Here's how the part is built. I have some questions about the finished solid (model axes, mm). Coordinates: 2 decimals unless noted, no trailing zeros. Write each loop counter-clockwise with the first axis right and the second up, starting at its lowest first coordinate (ties: lowest second). Pieces come first, ordered by that corner, then holes.
Item 1: If I drill on line 1 (Y direction, x = 50, z = 1.65); line 2 (Y direction, x = 68.5, z = 2.95); line 3 (Y direction, x = 30.5, z = 1.3), over which ranges is the centre line in solid material (lowest first)?
Item 2: If we section it at A-A (x = 26): Please give me the cut outline in (y, z) (3 decimals).
Item 3: If we section it at B-B (y = 26.5): Please give me the cut outline in (x, z) (3 decimals), then the cut area to 3 significant figures.
Item 4: We'd pull the mould along X, two halves only. Please class faces 1 (the face through (32.355, 36.9, 1.565)), 2 (the face through (48, 43, 0)): +X half, -X half, draft (parallel to the pull), parting line (faces both ways), or undercut.
Item 5: If we section it at C-C (y = 76): Please give me the cut outline in (x, z) (1 decimal), then the cut area to 3 significant figures.
Item 6: I'm going to push flat-ended pins straight in: pin 1 Ø0.6 at (x, z) = (69.5, 1.5) entering from +Y; pin 2 Ø1.5 at (x, z) = (33, 1) entering from -Y. Where does each tip first touch, or does it pass through?
from build123d import *

# Parameters (mm, degrees)
F1_DEPTH = 3.175
F2_R     = 38.1
F3_DEPTH = 3.175


with BuildPart() as f1:
    # F0 (on Top) → F1 (new body)
    with BuildSketch(Plane.XY):
        with BuildLine():
            ThreePointArc((22.616535, 24.245614), (30.63387, 30.737001), (40.389795, 34.089267))
            ThreePointArc((40.389795, 34.089267), (40.477862, 34.61335), (40.389795, 35.137434))
            ThreePointArc((40.389795, 35.137434), (45.513697, 36.794109), (50.780315, 37.917353))
            ThreePointArc((50.780315, 37.917353), (51.300846, 36.975201), (51.919628, 36.094457))
            ThreePointArc((51.919628, 36.094457), (52.978288, 35.400243), (54.243822, 35.433657))
            ThreePointArc((54.243822, 35.433657), (58.513462, 36.346899), (62.788658, 37.233766))
            ThreePointArc((62.788658, 37.233766), (65.134653, 35.56889), (67.573771, 34.043696))
            ThreePointArc((67.573771, 34.043696), (69.419666, 33.94496), (71.265139, 33.838619))
            ThreePointArc((71.265139, 33.838619), (70.692959, 34.529744), (70.103042, 35.205793))
            Line((70.103042, 35.205793), (68.029493, 35.205793))
            ThreePointArc((68.029493, 35.205793), (65.637095, 37.238695), (63.472249, 39.512392))
            ThreePointArc((63.472249, 39.512392), (60.923729, 39.08034), (58.345344, 38.897164))
            ThreePointArc((58.345344, 38.897164), (58.224015, 41.347541), (58.071908, 43.7962))
            ThreePointArc((58.071908, 43.7962), (57.696674, 45.899805), (56.499656, 47.669861))
            ThreePointArc((56.499656, 47.669861), (56.290628, 48.196762), (56.294583, 48.763596))
            ThreePointArc((56.294583, 48.763596), (56.786119, 49.19758), (57.069313, 49.788978))
            ThreePointArc((57.069313, 49.788978), (56.916742, 51.783508), (56.066722, 53.59428))
            ThreePointArc((56.066722, 53.59428), (55.232372, 51.877319), (55.337559, 49.971268))
            ThreePointArc((55.337559, 49.971268), (55.549432, 49.105391), (55.337559, 48.239514))
            ThreePointArc((55.337559, 48.239514), (47.307111, 47.375759), (39.615061, 44.912722))
            ThreePointArc((39.615061, 44.912722), (38.358176, 45.074826), (37.609871, 46.097606))
            ThreePointArc((37.609871, 46.097606), (37.734106, 50.78522), (38.065597, 55.462748))
            ThreePointArc((38.065597, 55.462748), (38.812979, 55.753921), (39.615061, 55.758972))
            ThreePointArc((39.615061, 55.758972), (41.209501, 55.956812), (41.916471, 57.399578))
            ThreePointArc((41.916471, 57.399578), (40.221037, 57.129852), (38.566899, 56.67042))
            ThreePointArc((38.566899, 56.67042), (38.216858, 57.049557), (38.18446, 57.564557))
            ThreePointArc((38.18446, 57.564557), (38.357401, 59.871413), (38.18446, 62.178269))
            ThreePointArc((38.18446, 62.178269), (37.440835, 64.224424), (35.951093, 65.811999))
            Line((35.951093, 65.811999), (35.632402, 65.254405))
            ThreePointArc((35.632402, 65.254405), (36.600109, 64.217879), (37.113506, 62.896036))
            ThreePointArc((37.113506, 62.896036), (37.228471, 61.99454), (37.131365, 61.090946))
            ThreePointArc((37.131365, 61.090946), (36.163108, 61.296761), (35.194539, 61.501101))
            ThreePointArc((35.194539, 61.501101), (33.947714, 62.86964), (32.567654, 64.1037))
            Line((32.567654, 64.1037), (32.203075, 63.625194))
            ThreePointArc((32.203075, 63.625194), (33.07375, 62.810062), (33.907115, 61.956823))
            ThreePointArc((33.907115, 61.956823), (34.294902, 61.413983), (33.872936, 60.897265))
            ThreePointArc((33.872936, 60.897265), (33.029886, 60.548272), (32.118395, 60.589653))
            ThreePointArc((32.118395, 60.589653), (31.306391, 61.318256), (30.63513, 62.178269))
            Line((30.63513, 62.178269), (30.181566, 61.751749))
            ThreePointArc((30.181566, 61.751749), (30.678242, 61.14598), (31.229733, 60.589653))
            ThreePointArc((31.229733, 60.589653), (31.298619, 60.339004), (31.229733, 60.088355))
            ThreePointArc((31.229733, 60.088355), (30.143393, 59.730613), (29.019469, 59.518699))
            ThreePointArc((29.019469, 59.518699), (28.791384, 59.23387), (29.019469, 58.949042))
            ThreePointArc((29.019469, 58.949042), (31.594216, 59.570867), (34.191944, 60.088355))
            ThreePointArc((34.191944, 60.088355), (35.476697, 60.240495), (36.698427, 59.814919))
            ThreePointArc((36.698427, 59.814919), (37.22257, 58.068271), (36.675639, 56.328624))
            ThreePointArc((36.675639, 56.328624), (32.654946, 55.750122), (28.734472, 54.686859))
            ThreePointArc((28.734472, 54.686859), (28.6864, 53.675594), (29.144622, 52.77282))
            ThreePointArc((29.144622, 52.77282), (31.110795, 52.387996), (33.109426, 52.248735))
            ThreePointArc((33.109426, 52.248735), (33.318546, 51.371466), (33.109426, 50.494198))
            ThreePointArc((33.109426, 50.494198), (31.960889, 46.614509), (31.240953, 42.632949))
            ThreePointArc((31.240953, 42.632949), (31.141519, 40.543829), (31.514391, 38.485851))
            ThreePointArc((31.514391, 38.485851), (32.367516, 36.877537), (33.268929, 35.295781))
            ThreePointArc((33.268929, 35.295781), (33.110196, 34.634594), (32.676484, 34.110896))
            ThreePointArc((32.676484, 34.110896), (25.940865, 29.887543), (19.916199, 24.700185))
            Line((19.916199, 24.700185), (22.616535, 24.245614))
        make_face()
    extrude(amount=F1_DEPTH)

    # F2 (on face) → F3 (join)
    with BuildSketch(Plane.XY.offset(3.175)):
        with Locations((45.590669, 45.256092)):
            Circle(F2_R)
        with BuildLine():
            ThreePointArc((69.788132, 24.700185), (47.34104, 13.554378), (23.803331, 22.161192))
            ThreePointArc((23.803331, 22.161192), (22.563249, 23.397446), (21.393206, 24.700185))
            ThreePointArc((21.393206, 24.700185), (34.640941, 75.058206), (77.340669, 45.256092))
            ThreePointArc((77.340669, 45.256092), (75.392782, 34.306365), (69.788132, 24.700185))
        make_face(mode=Mode.SUBTRACT)
        with BuildLine():
            ThreePointArc((23.803331, 22.161192), (23.149346, 23.168907), (22.616535, 24.245614))
            Line((22.616535, 24.245614), (22.616535, 24.700185))
            Line((22.616535, 24.700185), (21.393206, 24.700185))
            ThreePointArc((21.393206, 24.700185), (22.563249, 23.397446), (23.803331, 22.161192))
        make_face()
    extrude(amount=-F3_DEPTH)


solid = f1.part
Answer list:
1. line 1: y = 7.41 to 13.81, 37.79 to 47.85, 76.7 to 83.1
1. line 2: y = 14.81 to 23.27, 34 to 35.21, 67.24 to 75.7
1. line 3: y = 10.27 to 17.32, 30.66 to 32.9, 52.48 to 55.23, 59.32 to 59.83, 61.35 to 62.05, 73.19 to 80.24
2. outline: (12.579, 0) - (20.271, 0) - (20.271, 3.175) - (12.579, 3.175) - close; (27.562, 0) - (29.931, 0) - (29.931, 3.175) - (27.562, 3.175) - close; (70.241, 0) - (77.934, 0) - (77.934, 3.175) - (70.241, 3.175) - close
3. outline: (12.427, 0) - (19.973, 0) - (19.973, 3.175) - (12.427, 3.175) - close; (21.804, 0) - (24.795, 0) - (24.795, 3.175) - (21.804, 3.175) - close; (71.208, 0) - (78.754, 0) - (78.754, 3.175) - (71.208, 3.175) - close
3. area: 57.4 mm2
4. face 1: undercut
4. face 2: draft
5. outline: (23.1, 0) - (37.7, 0) - (37.7, 3.2) - (23.1, 3.2) - close; (53.5, 0) - (68.1, 0) - (68.1, 3.2) - (53.5, 3.2) - close
5. area: 92.5 mm2
6. pin 1: stops at y = 75.16
6. pin 2: stops at y = 9.04
